Geometry: final body of the model. Coordinates: model frame, mm. Round coordinates to 2 decimals unless told otherwise and drop trailing zeros. Loops run counter-clockwise (first coordinate to the right, second up) from the corner with the lowest first, then second, coordinate; pieces in that order, holes last. Notation, with made-up numbers: M 78.5,9 L 122.5,9 A15 cw 122.5,18 Z; hole C -9,-5.75 d3. An arc over 180 degrees is marked long. Write each question's results on one line, items separated by ' | '.
```python
from build123d import *


with BuildPart() as part:
    # Esquisse1 → Révolution1 (revolve)
    with BuildSketch(Plane.XY, mode=Mode.PRIVATE) as r_volution1_sk:
        with BuildLine():
            Line((12.631924887, 11), (18.631924887, 11))
            ThreePointArc((18.631924887, 11), (18.985478277, 10.853553391), (19.131924887, 10.5))
            Line((19.131924887, 10.5), (19.131924887, 8.5))
            Line((19.131924887, 8.5), (18.949161839, 8.5))
            Line((18.949161839, 8.5), (18.949161839, 8.804039909))
            Line((18.949161839, 8.804039909), (18.77636399, 8.804039909))
            Line((18.77636399, 8.804039909), (18.77636399, 8.5))
            Line((18.77636399, 8.5), (17.923212734, 8.5))
            ThreePointArc((17.923212734, 8.5), (15.631924887, 10), (13.340637039, 8.5))
            Line((13.340637039, 8.5), (12.487485783, 8.5))
            Line((12.487485783, 8.5), (12.487485783, 8.804039909))
            Line((12.487485783, 8.804039909), (12.314687935, 8.804039909))
            Line((12.314687935, 8.804039909), (12.314687935, 8.5))
            Line((12.314687935, 8.5), (12.131924887, 8.5))
            Line((12.131924887, 8.5), (12.131924887, 10.5))
            ThreePointArc((12.131924887, 10.5), (12.278371496, 10.853553391), (12.631924887, 11))
        make_face()
    revolve(r_volution1_sk.sketch.rotate(Axis((8.800669459, 0, 0), (1, 0, 0)), 90), axis=Axis((8.800669459, 0, 0), (1, 0, 0)))


solid = part.part
```
1. Section C-C (x = 15.5). Output: boundary loops of the cut face in (y, z).
Answer key:
outline: C 0,0 d22; hole C 0,0 d19.99
2. Pin query (flat end, axial travel): P1, Ø1, axis at x = 15, z = -1.5, coming from the +Y side; P2, Ø3, axis at x = 13, z = -4, coming from the -Y side; P3, Ø4, axis at x = 15, z = -6, coming from the +Y side. Return the tip coordinate at first contact, or that it passes through.
Answer key:
P1: stops at y = 10.95 | P2: stops at y = -10.71 | P3: stops at y = 10.25
3. Ray query, probe 1 along Y at (x, z) = (18.55, 0); probe 2 along Z at (x, y) = (16, 5.25); probe 3 along Y at (x, z) = (18.85, 0). Return the intervals inside material, ascending.
Answer key:
probe 1: y = -11 to -8.5, 8.5 to 11 | probe 2: z = -9.67 to -8.48, 8.48 to 9.67 | probe 3: y = -10.95 to -8.8, 8.8 to 10.95
4. Section D-D (x = 14.25). Output: boundary loops of the cut face in (y, z), then the cut area to 3 significant figures.
Answer key:
outline: C 0,0 d22; hole C 0,0 d19.17 | area: 91.6 mm²
5. Draft query along Z for faces 1 (the face through (18.344, -8.428, -1.107)), 2 (the face through (12.132, 0, -9)), 3 (the face through (15.67, 10.74, -2.38)). Return one class per face: pulls with the +Z half, pulls with the -Z half, needs draft (parallel to the pull), parting line crosses it, or undercut.
Answer key:
face 1: undercut | face 2: needs draft | face 3: parting line crosses it
